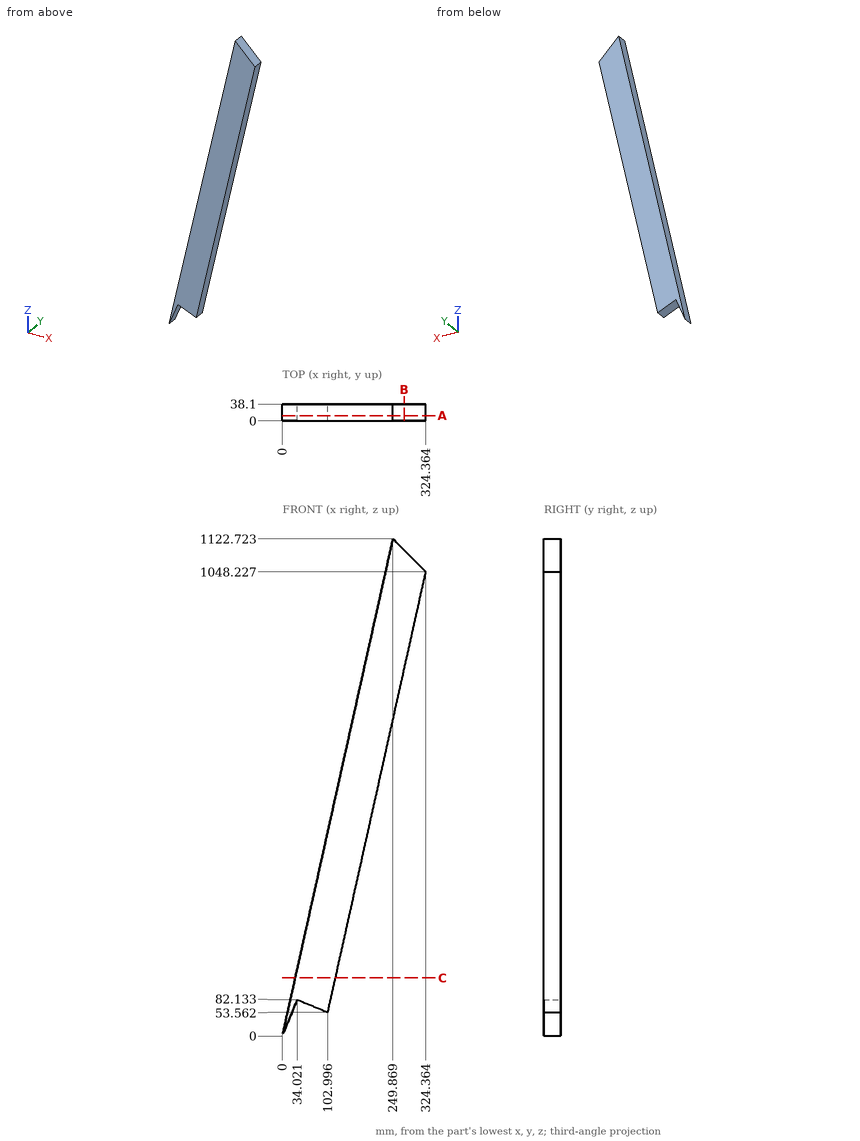
Study the drawing (mm; zero at the part's minimum x, y, z) and answer. Round coordinates to 2 decimals unless told otherwise and drop trailing zeros. Loops run counter-clockwise (first coordinate to the right, second up) from the corner with the lowest first, then second, coordinate; pieces in that order, holes last. Notation, with made-up numbers: (-20.75, 85) - (38.25, 85) arc R19 ccw to (38.25, 109) - close; hole circle Ø5 at (66, 8). An arc over 180 degrees is marked (long way). Use one line per item in the form item = value. Start each with the question number.
1. The part is cut by section B-B on x = 275.5. Determine the outline of the cut face in (y, z), then the cut area to 3 significant figures.
2. The part is cut by section A-A on y = 12. Determine the outline of the cut face in (x, z) (1 decimal), then the cut area to 3 significant figures.
3. Given pin 1 Ø2 at (y, z) = (25.5, 844.5) entering from +X; pin 2 Ø1.5 at (y, z) = (31.5, 605.5) entering from -X; pin 3 Ø10 at (y, z) = (32.5, 985) entering from +X (1 decimal), each flat-ended and moving along its own axis, determine where each tip first touches the part or whether it passes through.
4. The part is cut by section C-C on z = 131.5. Determine the outline of the cut face in (x, y), then the cut area to 3 significant figures.
5. Consider line 1 (X direction, y = 12, z = 110) (1 decimal); line 2 (X direction, y = 36.5, z = 860.5) (1 decimal). Determine where each line is inside the solid, lowest interval first. Write a range as [from, to].
Geometry check:
q1.outline = (0, 828.67) - (38.1, 828.67) - (38.1, 1097.09) - (0, 1097.09) - close
q1.area = 10,200 mm^2
q2.outline = (0, 0) - (34, 82.1) - (103, 53.6) - (324.4, 1048.2) - (249.9, 1122.7) - close
q2.area = 93,100 mm^2
q3.pin_1 = 279.25
q3.pin_2 = 134.59
q3.pin_3 = 311.4
q4.outline = (29.27, 0) - (120.34, 0) - (120.34, 38.1) - (29.27, 38.1) - close
q4.area = 3,470 mm^2
q5.line_1 = [24.5, 115.6]
q5.line_2 = [191.5, 282.6]
